Geometry check sheet. Reference: the model listing, model coordinates, mm. A direction names the side the tool comes from. Coordinates: 2 decimals unless noted, no trailing zeros. Loops run counter-clockwise (first coordinate to the right, second up) from the corner with the lowest first, then second, coordinate; pieces in that order, holes last.
from build123d import *

# Parameters (mm, degrees)
SKETCH_1_W          = 12
SKETCH_1_H          = 54
EXTRUDE_1_DEPTH     = 10
SKETCH_2_W          = 8
SKETCH_2_H          = 50
CUT_EXTRUDE_1_DEPTH = 10
SKETCH_3_W          = 13.565938191
SKETCH_3_H          = 57.788760324
CUT_EXTRUDE_2_DEPTH = 10
SKETCH_4_W          = 3
SKETCH_4_H          = 50
CUT_EXTRUDE_3_DEPTH = 1
FILLET_1_R          = 0.5


with BuildPart() as part:
    # 草圖1 → 填料-伸長1 (new body)
    with BuildSketch(Plane.XY):
        with Locations((-24.897904343, -6.146542517)):
            Rectangle(SKETCH_1_W, SKETCH_1_H)
    extrude(amount=EXTRUDE_1_DEPTH)

    # 草圖2 → 除料-伸長1 (cut)
    with BuildSketch(Plane.ZY.offset(30.897904343)):
        with Locations((4, -6.146542517)):
            Rectangle(SKETCH_2_W, SKETCH_2_H)
    extrude(amount=-CUT_EXTRUDE_1_DEPTH, mode=Mode.SUBTRACT)

    # 草圖3 → 除料-伸長2 (cut)
    with BuildSketch(Plane.ZY.offset(30.897904343)):
        with Locations((-1.782969096, -5.724817648)):
            Rectangle(SKETCH_3_W, SKETCH_3_H)
    extrude(amount=-CUT_EXTRUDE_2_DEPTH, mode=Mode.SUBTRACT)

    # 草圖4 → 除料-伸長3 (cut)
    with BuildSketch(Plane.ZY.offset(20.897904343)):
        with Locations((6.5, -6.146542517)):
            Rectangle(SKETCH_4_W, SKETCH_4_H)
    extrude(amount=-CUT_EXTRUDE_3_DEPTH, mode=Mode.SUBTRACT)

    # 圓角1
    fillet_1_edges = [part.edges().sort_by_distance(p)[0] for p in [
        (-24.897904343, 20.853457483, 10),
        (-30.897904343, -6.146542517, 10),
        (-30.897904343, -6.146542517, 8),
        (-30.897904343, 18.853457483, 6.5),
        (-30.897904343, -31.146542517, 6.5),
        (-19.897904343, 20.853457483, 0),
        (-19.897904343, -33.146542517, 0),
        (-24.897904343, -33.146542517, 10),
        (-18.897904343, -6.146542517, 0),
        (-19.897904343, -6.146542517, 8),
        (-19.897904343, -31.146542517, 6.5),
        (-19.897904343, -6.146542517, 5),
        (-19.897904343, 18.853457483, 6.5),
        (-20.897904343, -6.146542517, 5),
        (-30.897904343, -33.146542517, 7.5),
        (-30.897904343, 20.853457483, 7.5),
        (-18.897904343, 20.853457483, 5),
        (-18.897904343, -33.146542517, 5),
        (-18.897904343, -6.146542517, 10),
    ]]
    fillet(fillet_1_edges, radius=FILLET_1_R - 0.0001)  # a hair under: the kernel refuses the full size


solid = part.part
(1) Sectioned sample at B-B on x = -27.25. Record the cut outline in (y, z), and give its area (3 significant figures).
Findings:
outline: (-33.15, 5) - (-31.15, 5) - (-31.15, 8) - (18.85, 8) - (18.85, 5) - (20.85, 5) - (20.85, 9.5) arc R0.5 ccw to (20.35, 10) - (-32.65, 10) arc R0.5 ccw to (-33.15, 9.5) - close
area: 120 mm2
(2) Scan lines: L1, parallel to Z at x = -20.5, y = -14.5; L2, parallel to Y at x = -27, z = 6; L3, parallel to X at y = -31, z = 2.75. Record each from-to range of solid material in increasing order.
Findings:
L1: z = 0 to 4.99, 8 to 10
L2: y = -33.15 to -31.15, 18.85 to 20.85
L3: x = -20.9 to -18.9
(3) Access from +Z, -Z, +X, -X, +Y, -Y to the whole of each face (thin tool, end or side, straight path). Record for faces 1 (the flat face through (-30.898, -10, 9)), 2 (the flat face through (-26, -32, 5)).
Findings:
face 1: +Z, -Z, -X, +Y, -Y
face 2: -Z, -X, +Y, -Y
(4) Draft check along Z on faces 3 (the flat face through (-19.898, -6, 6)), 4 (the flat face through (-25, -33.147, 7)), 5 (the flat face through (-25, -6, 10)). Enter one of: +Z half, -Z half, draft (parallel to the pull), parting line (faces both ways), or undercut.
Findings:
face 3: undercut
face 4: draft
face 5: +Z half
(5) Gauge pin test, flat ends, axial feed: pin 1 Ø4 at (y, z) = (-6, 1.5) entering from -X; pin 2 Ø2 at (x, y) = (-28.5, 8) entering from -Z; pin 3 Ø1 at (x, y) = (-25, -32) entering from -Z. Record the tip position at first contact, or that the pin passes through.
Findings:
pin 1: stops at x = -20.9
pin 2: stops at z = 8
pin 3: stops at z = 5
(6) Sectioned sample at C-C on z = 1. Record the cut outline in (x, y).
Findings:
outline: (-20.9, -33.15) - (-19.4, -33.15) arc R0.5 ccw to (-18.9, -32.65) - (-18.9, 20.35) arc R0.5 ccw to (-19.4, 20.85) - (-20.9, 20.85) - close
